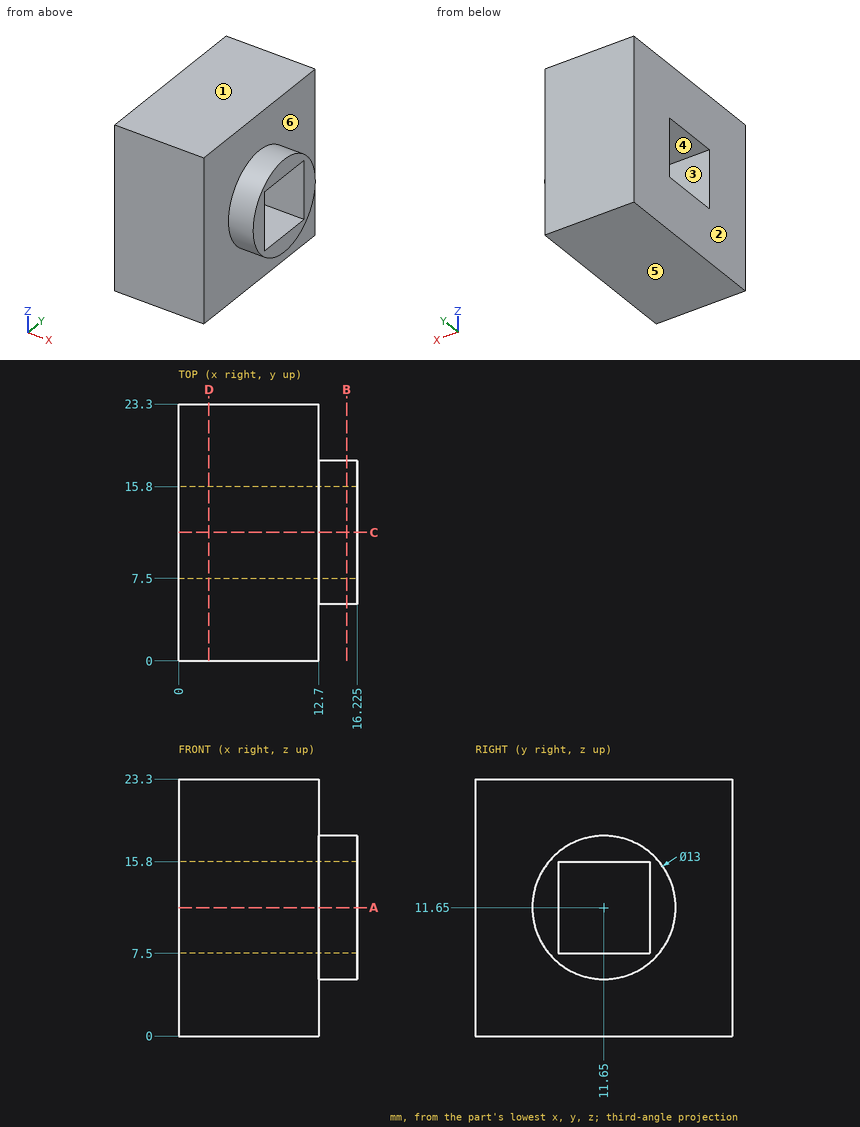
Design review of the part shown in the three views and the two pictorial views. Dimensions are in mm from the part's minimum x, y and z. A direction names the side the tool comes from. Give positions to 0.01 mm unless a question says otherwise; leave off trailing zeros. Write each loop counter-clockwise with the first axis right and the second up, starting at its lowest first coordinate (ties: lowest second). Pieces come first, ordered by that corner, then holes. Notation, with made-up numbers: (26, 7.5) - (46, 7.5) arc R33 ccw to (46, 46.5) - close; hole circle Ø6 at (62.5, 59). An arc over 180 degrees is marked (long way). Return JSON: item names as keys, results as strings. Group by question number.
(1) We need section D-D, the plane x = 2.75. Give the boundary of the cut face in (y, z).
(2) We need section B-B, the plane x = 15.25. Give the boundary of the cut face in (y, z).
(3) Insertion check: pin 1 (1.5 mm diameter, centred on y = 20.5, z = 9.5, fed in from +X). The pin has a flat end and moves straight along its axis. Give the tip position at first contact, or say it passes through.
(4) Machinability: for the marked faces 4, 5 and 6, which of the approach directions +Z, -Z, +X, -X, +Y, -Y give a long, thin tool a straight path to every point of the face, cutting with its end or side? Answer none if there is none.
(5) Mouldability with a two-part tool opening along Z and no side actions: class the marked faces 1, 2 and 3 as +Z half, -Z half, draft (parallel to the pull), parting line (faces both ways), or undercut.
(6) To check wall thickness, follow probe 1 along Y at (x, z) = (1.5, 15); probe 2 along X at (y, z) = (11.5, 3.5). State the ranges of each line that lie inside material, in increasing order.
(7) We need section A-A, the plane z = 11.65. Give the boundary of the cut face in (x, y) (3 decimals), then the cut area to 3 significant figures.
Reported:
{
 "1": {"outline": "(0, 0) - (23.3, 0) - (23.3, 23.3) - (0, 23.3) - close; hole (7.5, 7.5) - (15.8, 7.5) - (15.8, 15.8) - (7.5, 15.8) - close"},
 "2": {"outline": "circle Ø13 at (11.65, 11.65); hole (7.5, 7.5) - (15.8, 7.5) - (15.8, 15.8) - (7.5, 15.8) - close"},
 "3": {"pin 1": "stops at x = 12.7"},
 "4": {"face 4": "+X, -X", "face 5": "-Z, +X, -X, +Y, -Y", "face 6": "+X"},
 "5": {"face 1": "+Z half", "face 2": "draft", "face 3": "undercut"},
 "6": {"probe 1": "y = 0 to 7.5, 15.8 to 23.3", "probe 2": "x = 0 to 12.7"},
 "7": {"outline": "(0, 0) - (12.7, 0) - (12.7, 5.15) - (16.225, 5.15) - (16.225, 7.5) - (0, 7.5) - close; (0, 15.8) - (16.225, 15.8) - (16.225, 18.15) - (12.7, 18.15) - (12.7, 23.3) - (0, 23.3) - close", "area": "207 mm2"}
}
